Autodesk Inventor part; units mm, degrees
ref_plane "YZ Plane" through (0, 0, 0) normal (1, 0, 0) x (0, 1, 0)
ref_plane "XZ Plane" through (0, 0, 0) normal (0, 1, 0) x (-1, 0, 0)
ref_plane "XY Plane" through (0, 0, 0) normal (0, 0, 1) x (1, 0, 0)
sketch "Sketch1" plane through (0, 0, 0) normal (0, 0, 1) x (1, 0, 0)
  line L0 (-33.5, 4.5) -> (33.5, 4.5)
  line L1 (33.5, 4.5) -> (33.5, -4.5)
  line L2 (33.5, -4.5) -> (-33.5, -4.5)
  line L3 (-33.5, -4.5) -> (-33.5, 4.5)
  line L4 (-33.5, 4.5) -> (-41.5, 4.5)
  line L5 (-41.5, 4.5) -> (-41.5, -4.5)
  line L6 (-41.5, -4.5) -> (-33.5, -4.5)
  line L7 (-33.5, -4.5) -> (-33.5, 4.5)
  line L8 (33.5, 4.5) -> (41.5, 4.5)
  line L9 (41.5, 4.5) -> (41.5, -4.5)
  line L10 (41.5, -4.5) -> (33.5, -4.5)
  line L11 (33.5, -4.5) -> (33.5, 4.5)
  line L12 (-41.5, 0) -> (41.5, 0) construction
  circle A0 centre (-36.5, 0) radius 2.25
  circle A1 centre (36.5, 0) radius 2.25
  line L13 (0, 4.5) -> (0, -4.5) construction
  line L14 (-22.5, 4.5) -> (22.5, 4.5)
  line L15 (22.5, 4.5) -> (22.5, 6)
  line L16 (22.5, 6) -> (-22.5, 6)
  line L17 (-22.5, 6) -> (-22.5, 4.5)
  line L18 (-22.5, 6) -> (-41.5, 6)
  line L19 (-41.5, 6) -> (-41.5, 4.5)
  line L20 (-41.5, 4.5) -> (-22.5, 4.5)
  line L21 (-22.5, 4.5) -> (-22.5, 6)
  line L22 (22.5, 6) -> (41.5, 6)
  line L23 (41.5, 6) -> (41.5, 4.5)
  line L24 (41.5, 4.5) -> (22.5, 4.5)
  line L25 (22.5, 4.5) -> (22.5, 6)
  point P0 (0, 0)
  point P1 (0, 0)
  point P2 (0, 7)
  point P3 (0, 0)
  point P4 (0, 6)
  dimension "d0" = 9
  dimension "d1" = 67
  dimension "d2" = 4.5
  dimension "d3" = 4.5
  dimension "d4" = 5
  dimension "d5" = 3
  dimension "d6" = 5
  dimension "d7" = 3
  dimension "d12" = 45
  dimension "d13" = 1.5
  dimension "d29" = 83
extrude "Extrusion1" add sketch "Sketch1" along normal blind 1.5
extrude "Extrusion2" add sketch "Sketch1" along normal blind 30 contours L17 L16 L15 L0
sketch "Sketch2" plane through (-41.5, 4.5, 1.5) normal (0, -1, 0) x (1, 0, 0)
  line L0 (64, 0) -> (64, 28.5)
  line L1 (19, 28.5) -> (64, 28.5)
  line L2 (19, 0) -> (19, 28.5)
  circle A0 centre (23, 13.1) radius 5.5
  circle A1 centre (60, 13.1) radius 5.5
  line L3 (41.5, 28.5) -> (41.5, -1.5) construction
  line L4 (30.1, 23.5) -> (52.9, 23.5)
  line L5 (52.9, 23.5) -> (52.9, 2.7)
  line L6 (52.9, 2.7) -> (30.1, 2.7)
  line L7 (30.1, 2.7) -> (30.1, 23.5)
  line L8 (30.1, 13.1) -> (52.9, 13.1) construction
  point P0 (41.5, 23.5)
  dimension "d16" = 11
  dimension "d17" = 11
  dimension "d19" = 4
  dimension "d21" = 4
  dimension "d22" = 5
  dimension "d23" = 22.8
  dimension "d24" = 20.8
extrude "Extrusion3" cut sketch "Sketch2" against normal blind 10
fillet "Fillet1" radius 10 2 edges at (-22.5, 5.25, 30) (22.5, 5.25, 30)
fillet "Fillet2" radius 4 2 edges at (-41.5, -4.5, 0.75) (41.5, -4.5, 0.75)
properties part number "MotorBar"
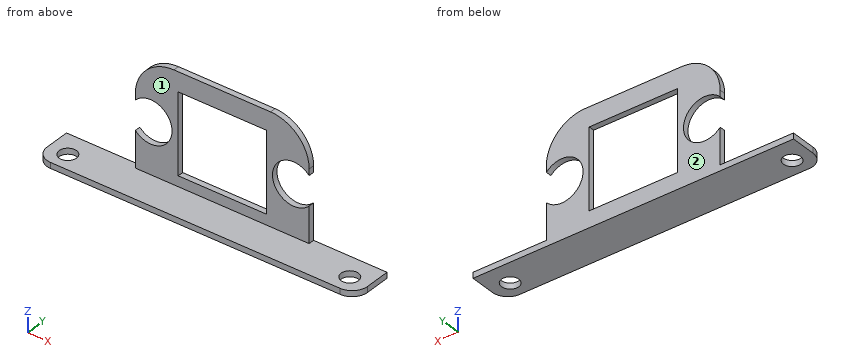
Can you work these out from the model? Positions are in its coordinate system, mm. Face numbers are marked on the shaded views. A direction names the side the tool comes from. Coordinates: 2 decimals unless noted, no trailing zeros. Loops run counter-clockwise (first coordinate to the right, second up) from the corner with the lowest first, then second, coordinate; pieces in that order, holes last. Notation, with made-up numbers: (-8.5, -24) -> (42.5, -24) arc R14 cw to (42.5, -20) -> close; hole circle Ø4 at (-28, 30). An arc over 180 degrees is marked (long way). Put each result on its own line as item: value. Start each with the question number.
Q1. I want a section at D-D (x = 36.5). Write out the boundary of the cut face in (y, z).
Q2. If I drill on line 1 (Y direction, x = 36.5, z = 0.85); line 2 (Z direction, x = 8, y = 4.75); line 3 (Z direction, x = 10, y = -0.5), over which ranges is the centre line in solid material (lowest first)? Write a range as [from, to].
Q3. I want a section at A-A (z = 14.6). Write out the boundary of the cut face in (x, y).
Q4. I want a section at B-B (x = -10). Write out the boundary of the cut face in (y, z), plus the area to 3 significant figures.
Q5. I'm going to push flat-ended pins straight in: P1, Ø1.2, axis at y = 5, z = 19.5, coming from the +X side; P2, Ø12.5, axis at x = -18.5, z = 14.6, coming from the -Y side; P3, Ø0.8, axis at x = 1.5, y = 5.5, coming from the -Z side; P4, Ø1.6, axis at y = 5, z = 6, coming from the -X side. Where does each tip first touch, or does it pass through?
Q6. I want a section at C-C (y = 1.5). Write out the boundary of the cut face in (x, z).
Q7. For the marked faces 1 and 2, which set-ups out of +Z, -Z, +X, -X, +Y, -Y let a thin tool reach every point of the face, with its end or its side?
Taken from the geometry:
1. outline: (-4.5, 0) -> (-2.25, 0) -> (-2.25, 1.5) -> (-4.5, 1.5) -> close; (2.25, 0) -> (6, 0) -> (6, 1.5) -> (2.25, 1.5) -> close
2. line 1: y = [-4.5, -2.25], [2.25, 6]
2. line 2: z = [0, 4.2], [25, 30]
2. line 3: z = [0, 1.5]
3. outline: (-13, 4.5) -> (-11.4, 4.5) -> (-11.4, 6) -> (-13, 6) -> close; (11.4, 4.5) -> (13, 4.5) -> (13, 6) -> (11.4, 6) -> close
4. outline: (-4.5, 0) -> (6, 0) -> (6, 4.2) -> (4.5, 4.2) -> (4.5, 1.5) -> (-4.5, 1.5) -> close; (4.5, 25) -> (6, 25) -> (6, 30) -> (4.5, 30) -> close
4. area: 27.3 mm2
5. P1: stops at x = 22.5
5. P2: stops at y = 4.5
5. P3: stops at z = 0
5. P4: stops at x = -22.5
6. outline: (-41.5, 0) -> (-38.18, 0) -> (-38.18, 1.5) -> (-41.5, 1.5) -> close; (-34.82, 0) -> (34.82, 0) -> (34.82, 1.5) -> (-34.82, 1.5) -> close; (38.18, 0) -> (41.5, 0) -> (41.5, 1.5) -> (38.18, 1.5) -> close
7. face 1: +Z, +X, -X, -Y
7. face 2: +Z, -Z, +X, -X, +Y
